```python
from build123d import *

# Parameters (mm, degrees)
SKETCH1_R               = 12
BOSS_EXTRUDE1_DEPTH     = 5
SKETCH2_R               = 12.5
BOSS_EXTRUDE2_DEPTH     = 1
SKETCH6_R               = 21.25
SKETCH6_R_2             = 18.5
SKETCH6_R_3             = 12.5
BOSS_EXTRUDE7_DEPTH     = 3
SKETCH6_3_R             = 21.25
SKETCH6_3_R_2           = 18.5
BOSS_EXTRUDE8_DEPTH     = 10
CUT_EXTRUDE2_DEPTH      = 35.045924866
CUT_EXTRUDE2_DEPTH_BACK = 35.045924866
SKETCH7_R               = 10
BOSS_EXTRUDE9_DEPTH     = 6
CIRPATTERN1_COUNT       = 4
SKETCH10_R              = 15.862399731
CUT_EXTRUDE3_DEPTH      = 1
CHAMFER1_SIZE           = 3
CHAMFER1_SIZE2          = 1.732050808
CHAMFER2_SIZE           = 0.7
CHAMFER2_SIZE2          = 1.435212689
FILLET1_R               = 1.2
FILLET2_R               = 1.5


with BuildPart() as part:
    # Sketch1 → Boss-Extrude1 (new body)
    with BuildSketch(Plane(origin=(0, 0, 0), x_dir=(1, 0, 0), z_dir=(0, 1, 0))):
        with Locations(Location((0, 0, 0), (0, 0, 270))):
            Circle(SKETCH1_R)
    extrude(amount=BOSS_EXTRUDE1_DEPTH)

    # Sketch2 → Boss-Extrude2 (add)
    with BuildSketch(Plane(origin=(0, 5, 0), x_dir=(1, 0, 0), z_dir=(0, 1, 0))):
        with Locations(Location((0, 0, 0), (0, 0, 270))):
            Circle(SKETCH2_R)
    extrude(amount=BOSS_EXTRUDE2_DEPTH)

    # Sketch6 → Boss-Extrude7 (add)
    # profile 1 of 3: a face of its own
    with BuildSketch(Plane(origin=(0, 6, 0), x_dir=(1, 0, 0), z_dir=(0, 1, 0))):
        with Locations(Location((0, 0, 0), (0, 0, 270))):
            Circle(SKETCH6_R)
        Circle(SKETCH6_R_2, mode=Mode.SUBTRACT)
    # profile 2 of 3: a face of its own
    with BuildSketch(Plane(origin=(0, 6, 0), x_dir=(1, 0, 0), z_dir=(0, 1, 0))):
        Circle(SKETCH6_R_2)
        with Locations(Location((0, 0, 0), (0, 0, 270))):
            Circle(SKETCH6_R_3, mode=Mode.SUBTRACT)
    # profile 3 of 3: a face of its own
    with BuildSketch(Plane(origin=(0, 6, 0), x_dir=(1, 0, 0), z_dir=(0, 1, 0))):
        with Locations(Location((0, 0, 0), (0, 0, 270))):
            Circle(SKETCH6_R_3)
    extrude(amount=BOSS_EXTRUDE7_DEPTH)

    # Sketch6<3> → Boss-Extrude8 (add)
    with BuildSketch(Plane(origin=(0, 6, 0), x_dir=(1, 0, 0), z_dir=(0, 1, 0))):
        with Locations(Location((0, 0, 0), (0, 0, 270))):
            Circle(SKETCH6_3_R)
        with Locations(Location((0, 0, 0), (0, 0, 270))):
            Circle(SKETCH6_3_R_2, mode=Mode.SUBTRACT)
    extrude(amount=BOSS_EXTRUDE8_DEPTH)

    # Sketch7 → Cut-Extrude2 (cut, two sides: drawn at the far end of the back side and taken through both)
    with BuildSketch(Plane.XZ.offset(-CUT_EXTRUDE2_DEPTH_BACK)):
        with Locations(Location((0, 0, 0), (0, 0, 90))):
            Circle(SKETCH7_R)
    extrude(amount=CUT_EXTRUDE2_DEPTH + CUT_EXTRUDE2_DEPTH_BACK, mode=Mode.SUBTRACT)

    # Sketch8 → Boss-Extrude9 (add)
    with BuildSketch(Plane(origin=(0, 9, 0), x_dir=(1, 0, 0), z_dir=(0, 1, 0))):
        with BuildLine():
            Line((17.165020759, 6.900149443), (15.300741035, 6.221944311))
            Line((15.300741035, 6.221944311), (14.239421514, 8.386472924))
            Line((14.239421514, 8.386472924), (16.043145314, 9.212355205))
            ThreePointArc((16.043145314, 9.212355205), (16.652877744, 8.079927373), (17.165020759, 6.900149443))
        make_face()
    boss_extrude9 = extrude(amount=BOSS_EXTRUDE9_DEPTH)

    # CirPattern1: Boss-Extrude9 ×4 about axis
    cirpattern1_axis = Axis((0, 0, 0), (0, 1, 0))
    for i in range(1, CIRPATTERN1_COUNT):
        add(boss_extrude9.rotate(cirpattern1_axis, i * 360 / CIRPATTERN1_COUNT))

    # Sketch10 → Cut-Extrude3 (cut)
    with BuildSketch(Plane(origin=(0, 9, 0), x_dir=(1, 0, 0), z_dir=(0, 1, 0))):
        with Locations(Location((0, 0, 0), (0, 0, 270))):
            Circle(SKETCH10_R)
    extrude(amount=-CUT_EXTRUDE3_DEPTH, mode=Mode.SUBTRACT)

    # Chamfer1
    chamfer1_edges = [part.edges().sort_by_distance(p)[0] for p in [
        (0, 8, -10),
    ]]
    chamfer1_side = [part.faces().sort_by_distance(p)[0] for p in [
        (0, 4, -10),
    ]]
    chamfer(chamfer1_edges, length=CHAMFER1_SIZE, length2=CHAMFER1_SIZE2, reference=chamfer1_side[0])

    # Chamfer2
    chamfer2_edges = [part.edges().sort_by_distance(p)[0] for p in [
        (0, 6, -12.5),
    ]]
    chamfer2_side = [part.faces().sort_by_distance(p)[0] for p in [
        (0, 5.5, -12.5),
    ]]
    chamfer(chamfer2_edges, length=CHAMFER2_SIZE, length2=CHAMFER2_SIZE2, reference=chamfer2_side[0])

    # Fillet1
    fillet1_edges = [part.edges().sort_by_distance(p)[0] for p in [
        (0, 8, -11.732050808),
        (0, 5, -10),
    ]]
    fillet(fillet1_edges, radius=FILLET1_R)

    # Fillet2
    fillet2_edges = [part.edges().sort_by_distance(p)[0] for p in [
        (0, 16, -21.25),
    ]]
    fillet(fillet2_edges, radius=FILLET2_R)


solid = part.part
```
Check sheet for the modelled part. Datum: model origin and axes. Units: mm. A direction names the side the tool comes from. Round coordinates to 2 decimals unless told otherwise and drop trailing zeros. Loops run counter-clockwise (first coordinate to the right, second up) from the corner with the lowest first, then second, coordinate; pieces in that order, holes last. Notation, with made-up numbers: (-10, -30) -> (13, -30) arc R34 cw to (13, 6) -> close; hole circle Ø3 at (21, -33.5). An arc over 180 degrees is marked (long way). Write item = value, one per line. Start each with the question number.
1) Gauge pin test, flat ends, axial feed: pin 1 Ø4 at (x, z) = (-13, -7.5) entering from -Y; pin 2 Ø1.5 at (x, y) = (-14.5, 13.5) entering from -Z; pin 3 Ø12 at (x, z) = (0, 0) entering from +Y; pin 4 Ø1.5 at (x, z) = (7.5, 16) entering from +Y. Record the tip position at first contact, or that the pin passes through.
2) Release check for a two-part mould opening along Z. For faces 4 (the flat face through (-14.778, 11.958, 7.289)), 5 (the flat face through (10, 5, -7)), 6 (the cylindrical face through (-11.09, 5.15, 5.77)) record: released by +Z, released by -Z, zero draft, split by the parting line, or undercut.
3) Thickness scan on probe 1 along X at (y, z) = (11, 0); probe 2 along X at (y, z) = (2.75, 0); probe 3 along Y at (x, z) = (15.5, -8.5). Record the ranges inside material, lowest first.
4) Sectioned sample at A-A, the plane y = 10.5. Record the cut outline in (x, z).
5) Sectioned sample at B-B, the plane y = 2.75. Record the cut outline in (x, z), plus the area to 3 significant figures.
6) Set-up check for faces 1 (the cylindrical face through (3.604, 2.465, 11.446)), 2 (the flat face through (8, 9, 14)), 3 (the flat face through (-6, 16, -18)): record each of +Z, -Z, +X, -X, +Y, -Y from which the full face is reachable in a straight line by a thin tool's end or side.
Results are:
q1.pin_1 = 5.55
q1.pin_2 = -16.2
q1.pin_3 = through
q1.pin_4 = 15
q2.face_4 = undercut
q2.face_5 = zero draft
q2.face_6 = split by the parting line
q3.probe_1 = -21.25 to -18.5, 18.5 to 21.25
q3.probe_2 = -12 to -10, 10 to 12
q3.probe_3 = 6 to 15
q4.outline = circle Ø42.5 at (0, 0); hole (-17.17, 6.9) arc R18.5 ccw to (-9.21, -16.04) -> (-8.39, -14.24) -> (-6.22, -15.3) -> (-6.9, -17.17) arc R18.5 ccw to (16.04, -9.21) -> (14.24, -8.39) -> (15.3, -6.22) -> (17.17, -6.9) arc R18.5 ccw to (9.21, 16.04) -> (8.39, 14.24) -> (6.22, 15.3) -> (6.9, 17.17) arc R18.5 ccw to (-16.04, 9.21) -> (-14.24, 8.39) -> (-15.3, 6.22) -> close
q5.outline = circle Ø24 at (0, 0); hole circle Ø20 at (0, 0)
q5.area = 138 mm^2
q6.face_1 = -Y
q6.face_2 = +Y
q6.face_3 = +Z, -Z, +X, -X, +Y
